from build123d import *

# Parameters (mm, degrees)
SKETCH1_W           = 238.125
SKETCH1_H           = 130.175
BOSS_EXTRUDE1_DEPTH = 203.2
SKETCH2_W           = 238.125
SKETCH2_H           = 130.175
CUT_EXTRUDE1_DEPTH  = 174.625
FILLET1_R           = 6.35


with BuildPart() as part:
    # Sketch1 → Boss-Extrude1 (new body)
    with BuildSketch(Plane.XY):
        Rectangle(SKETCH1_W, SKETCH1_H)
    extrude(amount=BOSS_EXTRUDE1_DEPTH)

    # Sketch2 → Cut-Extrude1 (cut)
    with BuildSketch(Plane(origin=(0, 0, 0), x_dir=(-1, 0, 0), z_dir=(0, 0, -1))):
        Rectangle(SKETCH2_W, SKETCH2_H)
        with BuildLine():
            ThreePointArc((114.3, -19.05), (82.938934322, -59.116688549), (36.5125, -38.297414599))
            ThreePointArc((36.5125, -38.297414599), (8.641725006, -59.410205821), (-25.430393972, -51.56031663))
            ThreePointArc((-25.430393972, -51.56031663), (-28.464210223, -57.798844223), (-34.925, -60.325))
            Line((-34.925, -60.325), (-104.775, -60.325))
            ThreePointArc((-104.775, -60.325), (-111.510192091, -57.535192091), (-114.3, -50.8))
            Line((-114.3, -50.8), (-114.3, -6.35))
            ThreePointArc((-114.3, -6.35), (-113.249567583, -2.001744111), (-110.329957107, 1.387446384))
            ThreePointArc((-110.329957107, 1.387446384), (-91.484237132, 55.967234316), (-36.5125, 38.297414599))
            ThreePointArc((-36.5125, 38.297414599), (-8.641725006, 59.410205821), (25.430393972, 51.56031663))
            ThreePointArc((25.430393972, 51.56031663), (28.464210223, 57.798844223), (34.925, 60.325))
            Line((34.925, 60.325), (104.775, 60.325))
            ThreePointArc((104.775, 60.325), (111.510192091, 57.535192091), (114.3, 50.8))
            Line((114.3, 50.8), (114.3, 6.35))
            ThreePointArc((114.3, 6.35), (113.249567583, 2.001744111), (110.329957107, -1.387446384))
            ThreePointArc((110.329957107, -1.387446384), (113.295260302, -9.998383558), (114.3, -19.05))
        make_face(mode=Mode.SUBTRACT)
    extrude(amount=-CUT_EXTRUDE1_DEPTH, mode=Mode.SUBTRACT)

    # Fillet1
    fillet1_edges = [part.edges().sort_by_distance(p)[0] for p in [
        (119.0625, -65.0875, 188.9125),
        (-119.0625, -65.0875, 188.9125),
        (-119.0625, 65.0875, 188.9125),
        (119.0625, 65.0875, 188.9125),
    ]]
    fillet(fillet1_edges, radius=FILLET1_R)


solid = part.part
Verification items for the finished model (mm, model axes). A direction names the side the tool comes from. Coordinates: 2 decimals unless noted, no trailing zeros. Order: outer loops, then holes, each group sorted by start corner. A loop starts at its lowest first (then second) coordinate and runs counter-clockwise, first axis right, second up. Notation, with made-up numbers: (47.5, -20) -> (73.5, -20) arc R17 ccw to (73.5, 8) -> close; hole circle Ø7 at (4, 61.25). An arc over 180 degrees is marked (long way). Use CSV: the item, a comma, the result in double quotes. Start each with the question number.
Q1. Draft check along X on faces 1 (the cylindrical face through (9.14, 59.3, 86.09)), 2 (the flat face through (114.3, -29, 86)), 3 (the flat face through (69, -60.325, 86)). Enter one of: +X half, -X half, draft (parallel to the pull), parting line (faces both ways), or undercut.
Q2. Tool access check on faces 4 (the cylindrical face through (-113.3, 2.1, 86.1)), 5 (the flat face through (36, 44, 174.625)), 6 (the flat face through (-69, 60.325, 86)). Record the directions out of +Z, -Z, +X, -X, +Y, -Y that give a thin tool (end or side, any length) a straight path to the whole face; none if there is none.
Q3. Section check A-A, the plane y = 19.05. Record the cut outline in (x, z) (1 decimal), and give its area (3 significant figures).
Q4. Section check D-D, the plane y = 43.5. Record the cut outline in (x, z) (1 decimal), and give its area (3 significant figures).
Q5. Section check C-C, the plane x = 96. Record the cut outline in (y, z) (1 decimal), and give its area (3 significant figures).
Q6. Thickness scan on line 1 along X through (y, z) = (21, 121); line 2 along Y through (x, z) = (0, 61.5) (3 decimals); line 3 along X through (y, z) = (-47, 38.5). Record the ranges inside material, lowest first.
Q7. Depth check by flat-ended pin: P1, Ø1.5, axis at x = -7, z = 170.5, coming from the -Y side; P2, Ø3, axis at y = -24, z = 118.5, coming from the -X side; P3, Ø8, axis at x = -6.5, z = 112, coming from the +Y side. Enter the tip coordinate at first touch or a pass-through.
Returned:
1,face 1,"undercut"
1,face 2,"+X half"
1,face 3,"draft"
2,face 4,"-Z, -X"
2,face 5,"-Z"
2,face 6,"-Z, +X, -X, +Y"
3,outline,"(-119.1, 174.6) -> (-114.3, 174.6) -> (-114.3, 0) -> (114.3, 0) -> (114.3, 174.6) -> (119.1, 174.6) -> (119.1, 203.2) -> (-119.1, 203.2) -> close"
3,area,"46,700 mm^2"
4,outline,"(-119.1, 174.6) -> (-114.3, 174.6) -> (-114.3, 0) -> (33.3, 0) -> (33.3, 174.6) -> (39.8, 174.6) -> (39.8, 0) -> (106.3, 0) -> (106.3, 174.6) -> (119.1, 174.6) -> (119.1, 203.2) -> (-119.1, 203.2) -> close"
4,area,"44,200 mm^2"
5,outline,"(-65.1, 174.6) -> (-60.3, 174.6) -> (-60.3, 0) -> (53.3, 0) -> (53.3, 174.6) -> (65.1, 174.6) -> (65.1, 203.2) -> (-65.1, 203.2) -> close"
5,area,"23,600 mm^2"
6,line 1,"x = -114.3 to 114.25"
6,line 2,"y = -60.325 to 60.325"
6,line 3,"x = -103.4 to -42.65, -30.37 to 114.3"
7,P1,"stops at y = -59.85"
7,P2,"stops at x = -114.16"
7,P3,"stops at y = 60.25"
